Job drawing, mm, ordinate dimensions from the low corner. One solid piece. Round coordinates to 2 decimals unless told otherwise and drop trailing zeros. Loops run counter-clockwise (first coordinate to the right, second up) from the corner with the lowest first, then second, coordinate; pieces in that order, holes last. Notation, with made-up numbers: M -33,31 L 15,31 A6 ccw 15,38 Z; hole C 39,-34 d7. An arc over 180 degrees is marked long. Use one line per item in the form item = value. Start each with the question number.
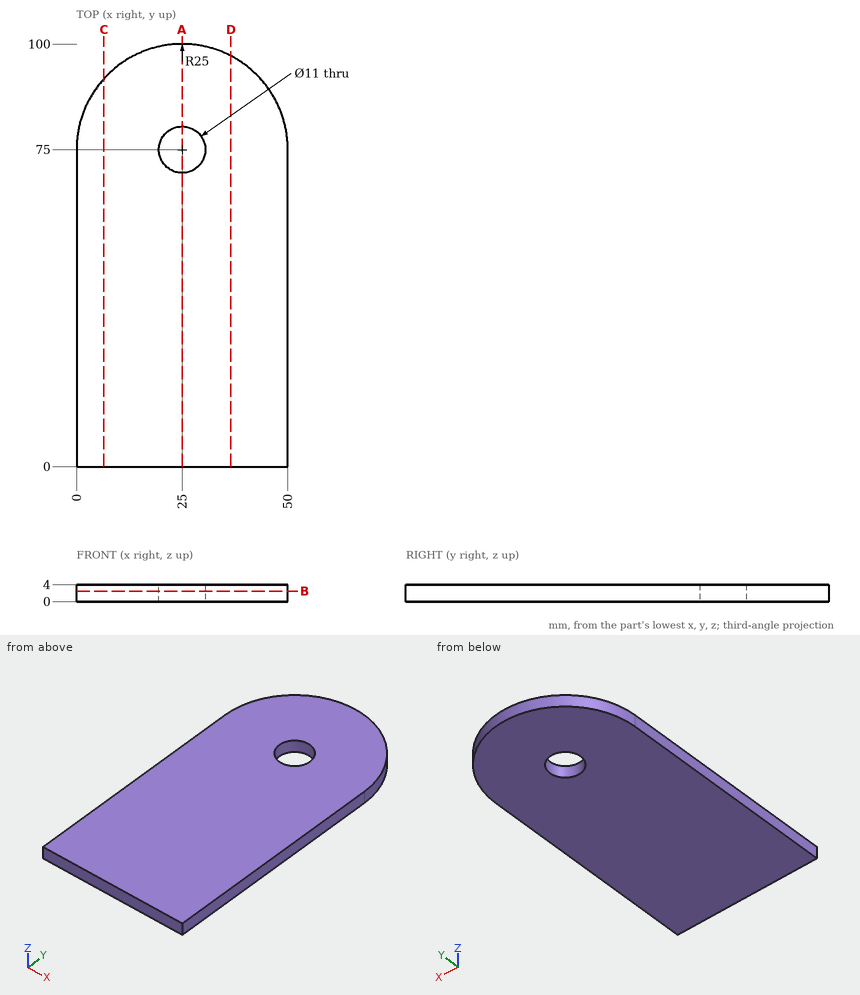
Q1. Wall check: probe 1 along Y at (x, z) = (25, 1.95); probe 2 along X at (y, z) = (78, 0.95); probe 3 along Y at (x, z) = (21, 2.45). Give the ranges that are in metal, low to high.
Q2. Saw through at C-C (x = 6.5). Give the cut face in (y, z), and give its area (3 significant figures).
Q3. Saw through at A-A (x = 25). Give the cut face in (y, z), and give its area (3 significant figures).
Q4. Saw through at B-B (z = 2.5). Give the cut face in (x, y), and give its area (3 significant figures).
Q5. Saw through at D-D (x = 36.5). Give the cut face in (y, z).
Filled in:
q1.probe_1 = 0 to 69.5, 80.5 to 100
q1.probe_2 = 0.18 to 20.39, 29.61 to 49.82
q1.probe_3 = 0 to 71.23, 78.77 to 99.68
q2.outline = M 0,0 L 91.82,0 L 91.82,4 L 0,4 Z
q2.area = 367 mm²
q3.outline = M 0,0 L 69.5,0 L 69.5,4 L 0,4 Z; M 80.5,0 L 100,0 L 100,4 L 80.5,4 Z
q3.area = 356 mm²
q4.outline = M 0,0 L 50,0 L 50,75 A25 ccw 0,75 Z; hole C 25,75 d11
q4.area = 4,640 mm²
q5.outline = M 0,0 L 97.2,0 L 97.2,4 L 0,4 Z
